Part model, mm, in its own coordinate system. A direction names the side the tool comes from. Coordinates: 2 decimals unless noted, no trailing zeros. Loops run counter-clockwise (first coordinate to the right, second up) from the corner with the lowest first, then second, coordinate; pieces in that order, holes last. Notation, with made-up numbers: (30.5, 81) -> (34.5, 81) arc R24 cw to (34.5, 98) -> close; hole circle Ø1 at (84, 54). An arc over 180 degrees is marked (long way). One line per item, written item: value. Start each with the question number.
from build123d import *

# Parameters (mm, degrees)
BOSS_EXTRUDE1_DEPTH         = 25.4
CUT_EXTRUDE1_DEPTH          = 112.462737913
F_1_4_20_TAPPED_HOLE1_D     = 5.1054
F_1_4_20_TAPPED_HOLE1_DEPTH = 16.51
F_1_4_20_TAPPED_HOLE1_TIP   = 1.533816902


with BuildPart() as part:
    # Sketch1 → Boss-Extrude1 (new body)
    with BuildSketch(Plane.XY):
        Polygon((0, 0), (-5.499261314, 9.525), (22.263261314, 9.525), (16.764, 0), (59.182, 0), (59.182, 38.16047619), (-42.418, 38.16047619), (-42.418, 0), align=None)
    extrude(amount=BOSS_EXTRUDE1_DEPTH)

    # Sketch2 → Cut-Extrude1 (cut, through all)
    with BuildSketch(Plane.ZY.offset(42.418)):
        Polygon((0, 38.16047619), (0, 25.46047619), (12.7, 38.16047619), align=None)
        Polygon((25.4, 38.16047619), (12.7, 38.16047619), (25.4, 25.46047619), align=None)
    extrude(amount=-CUT_EXTRUDE1_DEPTH, mode=Mode.SUBTRACT)

    # 1/4-20 Tapped Hole1
    with Locations(Plane(origin=(0, 38.16047619, 0), x_dir=(-1, 0, 0), z_dir=(0, 1, 0))):
        with Locations((29.718, 12.7), (-46.482, 12.7)):
            Hole(F_1_4_20_TAPPED_HOLE1_D / 2, depth=F_1_4_20_TAPPED_HOLE1_DEPTH)
            with Locations((0, 0, -(F_1_4_20_TAPPED_HOLE1_DEPTH + F_1_4_20_TAPPED_HOLE1_TIP / 2))):  # 118° drill point
                Cone(0, F_1_4_20_TAPPED_HOLE1_D / 2, F_1_4_20_TAPPED_HOLE1_TIP, mode=Mode.SUBTRACT)


solid = part.part
1) Tool access for faces 1 (the cylindrical face through (-27.36, 29.79, 11.72)), 2 (the flat face through (8, 9.525, 13)), 3 (the flat face through (8, 13, 0)): list every direction of +Z, -Z, +X, -X, +Y, -Y with a clear straight run to the whole face (end or side of a thin tool).
2) Pull direction Y, two halves, no side cores. Call faces 4 (the conical face through (46.24, 20.38, 13.07)), 5 (the flat face through (8, 13, 25.4)), 6 (the flat face through (-2.711, 4.696, 12.522)): +Y half, -Y half, draft (parallel to the pull), parting line (faces both ways), or undercut.
3) Slice it at A-A (y = 8). Give the cut face in (x, z), then the cut area to 3 significant figures.
4) Slice it at C-C (y = 28). Give the cut face in (x, z).
5) Pin check, flat tip, straight feed: pin 1 Ø1 at (x, z) = (12.5, 16) entering from -Y (3 decimals). Stop position of the tip, or through.
6) Slice it at D-D (z = 8.5). Give the cut face in (x, y) (3 decimals), then the cut area to 3 significant figures.
7) Probe line 1 (X direction, y = 26.5, z = 12.7); line 2 (Z direction, x = 46.5, y = 22.5); line 3 (Y direction, x = -3, z = 12.75) (3 decimals). List the from-to ranges inside material, lowest first. Write a range as from..to.
8) Slice it at B-B (x = 34). Give the cut face in (y, z), then the cut area to 3 significant figures.
Check sheet entries:
1. face 1: +Y
1. face 2: +Z, -Z
1. face 3: -Z, +X, -X, +Y, -Y
2. face 4: +Y half
2. face 5: draft
2. face 6: undercut
3. outline: (-42.42, 0) -> (-4.62, 0) -> (-4.62, 25.4) -> (-42.42, 25.4) -> close; (21.38, 0) -> (59.18, 0) -> (59.18, 25.4) -> (21.38, 25.4) -> close
3. area: 1,920 mm^2
4. outline: (-42.42, 2.54) -> (59.18, 2.54) -> (59.18, 22.86) -> (-42.42, 22.86) -> close; hole circle Ø5.11 at (-29.72, 12.7); hole circle Ø5.11 at (46.48, 12.7)
5. pin 1: stops at y = 9.525
6. outline: (-42.418, 0) -> (0, 0) -> (-5.499, 9.525) -> (22.263, 9.525) -> (16.764, 0) -> (59.182, 0) -> (59.182, 33.96) -> (-42.418, 33.96) -> close
6. area: 3,240 mm^2
7. line 1: x = -42.42..-32.27, -27.17..43.93, 49.03..59.18
7. line 2: z = 0..10.15, 15.25..25.4
7. line 3: y = 0..5.196, 9.525..38.11
8. outline: (0, 0) -> (25.46, 0) -> (38.16, 12.7) -> (25.46, 25.4) -> (0, 25.4) -> close
8. area: 808 mm^2
